Study the drawing (mm; zero at the part's minimum x, y, z) and answer. A direction names the side the tool comes from. Round coordinates to 2 decimals unless told otherwise and drop trailing zeros. Order: outer loops, then holes, each group sorted by start corner. A loop starts at its lowest first (then second) coordinate and runs counter-clockwise, first axis right, second up. Notation, with made-up numbers: (4.5, 7) -> (42.5, 7) arc R22 ccw to (42.5, 35) -> close; hole circle Ø10 at (-13, 31). An arc over 180 degrees is marked (long way). Answer in a Markdown table with one row per item. Add a question column.
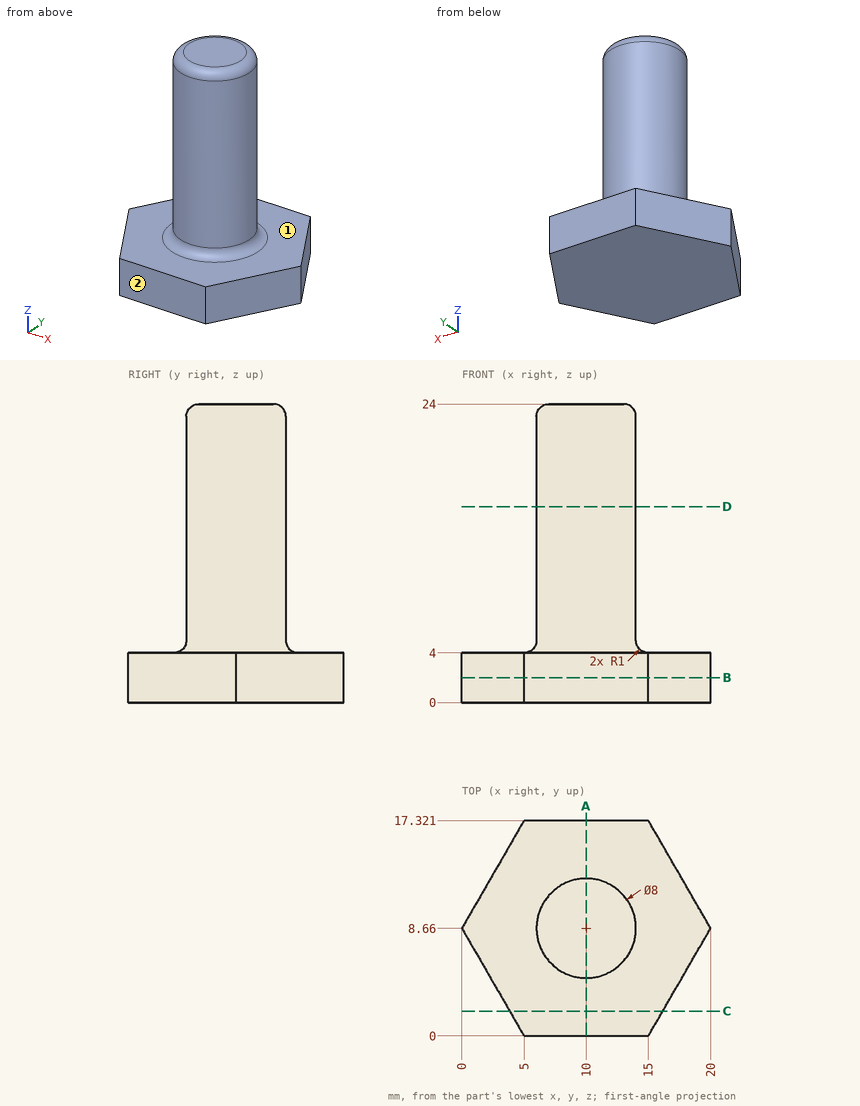
Item 1: Find the intervals of material crossed by probe 1 along X at (y, z) = (8.5, 17.75); probe 2 along Z at (x, y) = (15, 7.25); probe 3 along X at (y, z) = (5.75, 5.25) (1 decimal), in increasing order. Write a range as [from, to].
Item 2: A tool of negligible diameter and unlimited length cuts with its end or side. For the marked faces 1 and 2, from which of +Z, -Z, +X, -X, +Y, -Y can it reach the whole face along a straight path? Write none if from no direction.
Item 3: The part is cut by section A-A, the plane x = 10. Give the vertices of the cut face in (y, z).
Item 4: The part is cut by section C-C, the plane y = 2. Give the vertices of the cut face in (x, z) (1 decimal).
Item 5: Flat-ended cylindrical pins translate along their axes: P1, Ø6, axis at x = 4.5, y = 5, coming from the -Z side; P2, Ø12, axis at x = 11, z = 20, coming from the +Y side; P3, Ø6, axis at x = 3.5, z = 11.5, coming from the -Y side (1 decimal); P4, Ø10, axis at y = 15.5, z = 16, coming from the +X side. Find the tip coordinate at first contact, or state that the pin passes through.
Item 6: The part is cut by section B-B, the plane z = 2. Give the vertices of the cut face in (x, y).
Item 7: The part is cut by section D-D, the plane z = 15.75. Give the vertices of the cut face in (x, y).
Resolved:
| question | item | result |
|---|---|---|
| 1 | probe 1 | [6, 14] |
| 1 | probe 2 | [0, 4] |
| 1 | probe 3 | [7.3, 12.7] |
| 2 | face 1 | +Z |
| 2 | face 2 | +Z, -Z, +X, -X, -Y |
| 3 | outline | (0, 0) -> (17.32, 0) -> (17.32, 4) -> (13.66, 4) arc R1 cw to (12.66, 5) -> (12.66, 23) arc R1 ccw to (11.66, 24) -> (5.66, 24) arc R1 ccw to (4.66, 23) -> (4.66, 5) arc R1 cw to (3.66, 4) -> (0, 4) -> close |
| 4 | outline | (3.8, 0) -> (16.2, 0) -> (16.2, 4) -> (3.8, 4) -> close |
| 5 | P1 | z = 0 |
| 5 | P2 | y = 12.66 |
| 5 | P3 | y = 6.7 |
| 5 | P4 | x = 13.55 |
| 6 | outline | (0, 8.66) -> (5, 0) -> (15, 0) -> (20, 8.66) -> (15, 17.32) -> (5, 17.32) -> close |
| 7 | outline | circle Ø8 at (10, 8.66) |
